from build123d import *

# Parameters (mm, degrees)
F1_DEPTH = 6.35
F3_DEPTH = 4.191


with BuildPart() as f1:
    # F0 (on Right) → F1 (new body)
    with BuildSketch(Plane.YZ):
        with BuildLine():
            Line((24.892, -3.5873989895), (3.2653610572, 14.559505771))
            ThreePointArc((3.2653610572, 14.559505771), (1.7374623281, 15.4416385136), (0, 15.748))
            ThreePointArc((0, 15.748), (-1.7374623281, 15.4416385136), (-3.2653610572, 14.559505771))
            Line((-3.2653610572, 14.559505771), (-24.892, -3.5873989895))
            Line((-24.892, -3.5873989895), (-24.892, -11.0821703985))
            Line((-24.892, -11.0821703985), (-2.1469007696, -0.4759564419))
            ThreePointArc((-2.1469007696, -0.4759564419), (-1.0995132388, -0.1204162838), (0, 0))
            ThreePointArc((0, 0), (1.0995132388, -0.1204162838), (2.1469007696, -0.4759564419))
            Line((2.1469007696, -0.4759564419), (24.892, -11.0821703985))
            Line((24.892, -11.0821703985), (24.892, -3.5873989895))
        make_face()
    extrude(amount=F1_DEPTH)

    # F2 (on face) → F3 (cut)
    with BuildSketch(Plane.YZ.offset(6.35)):
        Polygon((22.098, -9.7793068016), (24.892, -11.0821703985), (24.892, -3.5873989895), (22.098, -1.2429546199), align=None)
        Polygon((-22.098, -9.7793068016), (-22.098, -1.2429546199), (-24.892, -3.5873989895), (-24.892, -11.0821703985), align=None)
    extrude(amount=-F3_DEPTH, mode=Mode.SUBTRACT)


solid = f1.part
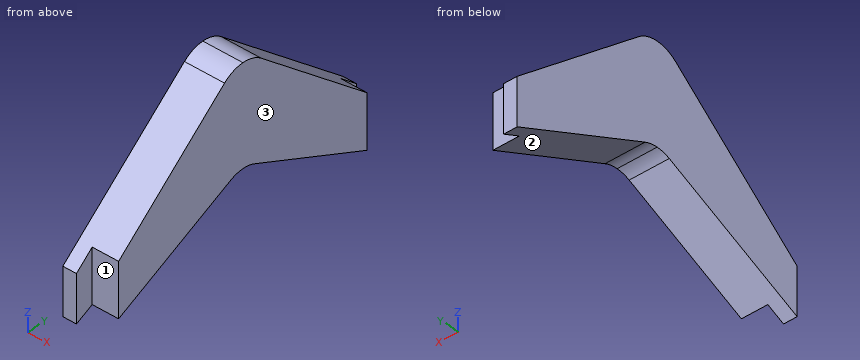
Model file for the job. Use its own axes, mm. Face numbers are marked on the shaded views. A direction names the side the tool comes from. Give positions to 0.01 mm unless a question says otherwise; leave off trailing zeros. Write each loop counter-clockwise with the first axis right and the second up, starting at its lowest first coordinate (ties: lowest second). Pieces come first, ordered by that corner, then holes. Notation, with made-up numbers: M 1,24.5 L 48,24.5 A21 cw 48,38.5 Z; hole C 63.5,-19 d1. An arc over 180 degrees is marked long. One line per item, written item: value. Start each with the question number.
Q1. Saw through at D-D, the plane z = -7.5. Write the cut outline in (x, y), plus the area to 3 significant figures.
Q2. Probe probe 1 along Y at (x, z) = (4.75, -1.5); probe 2 along Y at (x, z) = (6, -3.75); probe 3 along Z at (x, y) = (1.5, 14). List the from-to ranges inside material, lowest first. Write a range as [from, to].
Q3. Saw through at C-C, the plane y = -19. Write the cut outline in (x, z).
Q4. Saw through at B-B, the plane z = -4.5. Write the cut outline in (x, y), plus the area to 3 significant figures.
Q5. Saw through at A-A, the plane x = 3.25. Write the cut outline in (y, z), plus the area to 3 significant figures.
Q6. 3-axis set-ups, long thin cutter, end or side, ignore diameter. For the marked faces 1, 2 and 3: which of +Z, -Z, +X, -X, +Y, -Y reach the whole face in a straight line?
Q7. Drop flat-ended pins along their axis: pin 1 Ø3 at (x, z) = (3, -1.5) entering from -Y; pin 2 Ø1 at (x, z) = (5.5, 9) entering from +Y; pin 3 Ø1.5 at (x, z) = (4, 1.5) entering from +Y. Give the stop position or say it passes through.
Output values:
1. outline: M 0,-24.89 L 2.16,-24.89 L 2.16,-22.1 L 6.35,-22.1 L 6.35,-17.21 L 0,-17.21 Z; M 0,17.21 L 6.35,17.21 L 6.35,22.1 L 2.16,22.1 L 2.16,24.89 L 0,24.89 Z
1. area: 74.1 mm²
2. probe 1: y = [-22.1, -4.34], [4.34, 22.1]
2. probe 2: y = [-22.1, -9.17], [9.17, 22.1]
2. probe 3: z = [-6, 5.55]
3. outline: M 0,-8.33 L 6.35,-8.33 L 6.35,1.36 L 0,1.36 Z
4. outline: M 0,-24.89 L 2.16,-24.89 L 2.16,-22.1 L 6.35,-22.1 L 6.35,-10.78 L 0,-10.78 Z; M 0,10.78 L 6.35,10.78 L 6.35,22.1 L 2.16,22.1 L 2.16,24.89 L 0,24.89 Z
4. area: 156 mm²
5. outline: M -22.1,-9.78 L -2.15,-0.48 A5.08 cw 2.15,-0.48 L 22.1,-9.78 L 22.1,-1.24 L 3.27,14.56 A5.08 ccw -3.27,14.56 L -22.1,-1.24 Z
5. area: 556 mm²
6. face 1: +Z, -Z, +X, -Y
6. face 2: -Z, +X, -X
6. face 3: +Z, -Z, +X, +Y, -Y
7. pin 1: stops at y = -23.88
7. pin 2: stops at y = 10.49
7. pin 3: stops at y = 19.72
